Work out the finished part from the listing and answer in its coordinate system (mm). Round coordinates to 2 decimals unless told otherwise and drop trailing zeros. Write each loop counter-clockwise with the first axis right and the second up, starting at its lowest first coordinate (ties: lowest second). Pieces come first, ordered by that corner, then holes.
from build123d import *

# Parameters (mm, degrees)
SKETCH_1_R          = 10
EXTRUDE_1_DEPTH     = 608
SKETCH_2_R          = 2.75
CUT_EXTRUDE_2_DEPTH = 450


with BuildPart() as part:
    # 草图1 → 凸台-拉伸1 (new body)
    with BuildSketch(Plane.XY):
        with Locations((0, 27)):
            Circle(SKETCH_1_R)
        with BuildLine():
            Line((-22.5, 5), (-22.5, 0))
            Line((-22.5, 0), (0, 0))
            Line((0, 0), (0, 17))
            ThreePointArc((0, 17), (-1.870828693, 17.176558648), (-3.67559519, 17.7))
            Line((-3.67559519, 17.7), (-4, 17.7))
            Line((-4, 17.7), (-9.5, 10))
            Line((-9.5, 10), (-9.5, 5))
            Line((-9.5, 5), (-22.5, 5))
        make_face()
        with BuildLine():
            Line((0, 17), (0, 0))
            Line((0, 0), (22.5, 0))
            Line((22.5, 0), (22.5, 5))
            Line((22.5, 5), (9.5, 5))
            Line((9.5, 5), (9.5, 10))
            Line((9.5, 10), (4, 17.7))
            Line((4, 17.7), (3.67559519, 17.7))
            ThreePointArc((3.67559519, 17.7), (1.870828693, 17.176558648), (0, 17))
        make_face()
    extrude(amount=EXTRUDE_1_DEPTH)

    # 草图2 → 切除-拉伸2 (cut)
    with BuildSketch(Plane(origin=(0, 0, 0), x_dir=(1, 0, 0), z_dir=(0, 1, 0))):
        with Locations((15, -304)):
            Circle(SKETCH_2_R)
        with Locations((15, -454)):
            Circle(SKETCH_2_R)
        with Locations(Location((-15, -304, 0), (0, 0, 180))):
            Circle(SKETCH_2_R)
        with Locations(Location((-15, -454, 0), (0, 0, 180))):
            Circle(SKETCH_2_R)
        with Locations((15, -154)):
            Circle(SKETCH_2_R)
        with Locations(Location((-15, -154, 0), (0, 0, 180))):
            Circle(SKETCH_2_R)
    extrude(amount=CUT_EXTRUDE_2_DEPTH, mode=Mode.SUBTRACT)


solid = part.part
Q1. Find section A-A (y = 27). Determine the outline of the cut face in (x, z), plus the area to 3 significant figures.
Q2. Find the intervals of material crossed by L1, parallel to Z at x = -15, y = 3.25; L2, parallel to X at y = 3.3, z = 154; L3, parallel to Y at x = 18, z = 354, in increasing order.
Q3. Given pin 1 (5 mm diameter, centred on x = -15, z = 454, fed in from +Y); pin 2 (1.5 mm diameter, centred on y = 29, z = 205, fed in from -X); pin 3 (1.5 mm diameter, centred on y = 8, z = 455, fed in from +X); pin 4 (10.5 mm diameter, centred on x = -17.5, z = 371, fed in from +Y), each flat-ended and moving along its own axis, determine where each tip first touches the part or whether it passes through.
Q4. The mould has two halves that part along Y. Classify faces 1 (the face through (0, 15, 608)), 2 (the face through (0, 0, 300)), 3 (the face through (0, 37, 300)): +Y half, -Y half, draft (parallel to the pull), parting line (faces both ways), or undercut.
Report:
1. outline: (-10, 0) - (10, 0) - (10, 608) - (-10, 608) - close
1. area: 12,200 mm2
2. L1: z = 0 to 151.25, 156.75 to 301.25, 306.75 to 451.25, 456.75 to 608
2. L2: x = -22.5 to -17.75, -12.25 to 12.25, 17.75 to 22.5
2. L3: y = 0 to 5
3. pin 1: passes through
3. pin 2: stops at x = -9.92
3. pin 3: stops at x = 9.5
3. pin 4: stops at y = 5
4. face 1: draft
4. face 2: -Y half
4. face 3: undercut
